from build123d import *

# Parameters (mm, degrees)
SKETCH1_W                 = 20.32
SKETCH1_H                 = 20.32
BOSS_EXTRUDE1_DEPTH       = 6.985
SKETCH5_W                 = 22.86
SKETCH5_H                 = 0.635
CUT_EXTRUDE3_DEPTH        = 1
CUT_EXTRUDE3_DEPTH_BACK   = 7.985
F_6_CLEARANCE_HOLE1_D     = 3.7973
F_6_CLEARANCE_HOLE1_DEPTH = 6.985
FILLET1_R                 = 2.54
F_8_0MM_DOWEL_HOLE1_D     = 8
F_8_0MM_DOWEL_HOLE1_DEPTH = 6.985
F_6_CLEARANCE_HOLE2_D     = 3.7973


with BuildPart() as part:
    # Sketch1 → Boss-Extrude1 (new body)
    with BuildSketch(Plane.XY):
        Rectangle(SKETCH1_W, SKETCH1_H)
    extrude(amount=BOSS_EXTRUDE1_DEPTH)

    # Sketch5 → Cut-Extrude3 (cut, two sides)
    with BuildSketch(Plane.XY.offset(6.985)) as cut_extrude3_sk:
        with Locations((-15.137429848, 0.144302155)):
            Rectangle(SKETCH5_W, SKETCH5_H)
    extrude(amount=CUT_EXTRUDE3_DEPTH, mode=Mode.SUBTRACT)
    extrude(cut_extrude3_sk.sketch, amount=-CUT_EXTRUDE3_DEPTH_BACK, mode=Mode.SUBTRACT)

    # #6 Clearance Hole1
    with Locations(Plane.XY.offset(6.985)):
        with Locations((6.914797213, 6.914797213), (6.914797213, -6.914797213)):
            Hole(F_6_CLEARANCE_HOLE1_D / 2, depth=F_6_CLEARANCE_HOLE1_DEPTH)

    # Fillet1
    fillet1_edges = [part.edges().sort_by_distance(p)[0] for p in [
        (10.16, -10.16, 3.4925),
        (-10.16, -10.16, 3.4925),
        (-10.16, 10.16, 3.4925),
        (10.16, 10.16, 3.4925),
    ]]
    fillet(fillet1_edges, radius=FILLET1_R)

    # Ø8.0mm Dowel Hole1
    with Locations(Plane.XY.offset(6.985)):
        with Locations((0, 0)):
            Hole(F_8_0MM_DOWEL_HOLE1_D / 2, depth=F_8_0MM_DOWEL_HOLE1_DEPTH)

    # #6 Clearance Hole2 (through all)
    with Locations(Plane(origin=(0, 10.16, 0), x_dir=(1, 0, 0), z_dir=(0, 1, 0))):
        with Locations((-6.096, -3.81)):
            Hole(F_6_CLEARANCE_HOLE2_D / 2)


solid = part.part
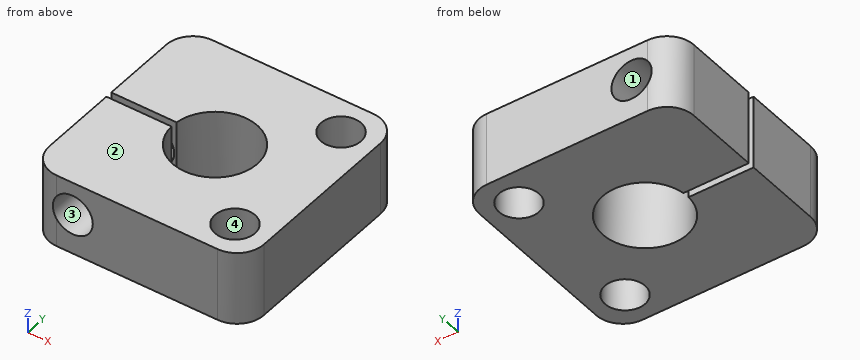
Source: CAD feature listing. Evaluate the final solid. Frame: model axes, mm. Face numbers are marked on the shaded views. Give positions to 0.01 mm unless a question says otherwise; leave off trailing zeros. Write each loop counter-clockwise with the first axis right and the second up, starting at its lowest first coordinate (ties: lowest second). Pieces come first, ordered by that corner, then holes. Notation, with made-up numbers: M 15.5,-33.75 L 45.5,-33.75 A24 cw 45.5,2.25 Z; hole C -39.5,17.25 d10. An arc over 180 degrees is marked long. Answer as a JSON object with one key per item and string values.
Q1. Cut plane B-B, the plane z = 4.5. Return the cut outline in (x, y).
Geometry check:
{"outline": "M -10.16,-7.62 A2.54 ccw -7.86,-10.15 L -7.86,-0.17 L -10.16,-0.17 Z; M -10.16,0.46 L -7.86,0.46 L -7.86,10.15 A2.54 ccw -10.16,7.62 Z; M -4.33,-10.16 L 7.62,-10.16 A2.54 ccw 10.16,-7.62 L 10.16,7.62 A2.54 ccw 7.62,10.16 L -4.33,10.16 L -4.33,0.46 L -3.97,0.46 A4 cw long -4,-0.17 L -4.33,-0.17 Z; hole C 6.91,-6.91 d3.8; hole C 6.91,6.91 d3.8"}
Q2. Ray query, line 1 along Y through (x, z) = (0, 3.75); line 2 along Y through (x, z) = (7.25, 2); line 3 along Y through (x, z) = (-4.5, 2.25). Return the intervals inside material, ascending.
Geometry check:
{"line 1": "y = -10.16 to -4, 4 to 10.16", "line 2": "y = -10.16 to -8.78, -5.05 to 5.05, 8.78 to 10.16", "line 3": "y = -10.16 to -0.17, 0.46 to 10.16"}
Q3. Cut plane C-C, the plane y = 1.75. Return the cut outline in (x, z) (3 decimals).
Geometry check:
{"outline": "M -10.16,0 L -3.597,0 L -3.597,6.985 L -10.16,6.985 Z; M 3.597,0 L 10.16,0 L 10.16,6.985 L 3.597,6.985 Z; hole C -6.096,3.81 d3.797"}
Q4. Mould query, pull axis Z, two halves, no side actions, for the marked faces 1, 2, 3 and 4. Classes: +Z half, -Z half, draft (parallel to the pull), parting line (faces both ways), or undercut.
Geometry check:
{"face 1": "undercut", "face 2": "+Z half", "face 3": "undercut", "face 4": "draft"}
Q5. Cut plane A-A, the plane x = 0. Return the cut outline in (y, z) (3 decimals).
Geometry check:
{"outline": "M -10.16,0 L -4,0 L -4,6.985 L -10.16,6.985 Z; M 4,0 L 10.16,0 L 10.16,6.985 L 4,6.985 Z"}
Q6. Cut plane D-D, the plane y = 4.25. Return the cut outline in (x, z) (3 decimals).
Geometry check:
{"outline": "M -10.16,0 L 10.16,0 L 10.16,6.985 L -10.16,6.985 Z; hole C -6.096,3.81 d3.797"}
